Check sheet for the modelled part. Datum: model origin and axes. Units: mm. A direction names the side the tool comes from. Give positions to 0.01 mm unless a question says otherwise; leave off trailing zeros. Order: outer loops, then holes, each group sorted by start corner. A loop starts at its lowest first (then second) coordinate and runs counter-clockwise, first axis right, second up. Notation, with made-up numbers: (85.25, 30) -> (90.25, 30) arc R11 ccw to (90.25, 42) -> close; hole circle Ø5 at (58, 63). An arc over 180 degrees is marked (long way). One line per question, with ' | ' between items.
```python
from build123d import *

# Parameters (mm, degrees)
F1_DEPTH = 152.4
F2_DEPTH = 12.7
F3_R     = 3.175
F4_R     = 1.5875
F5_R     = 3.175
F6_DEPTH = 25.4


# Not quite as in the source:
# - a feature names something its author has since deleted; it is built from what else it names


with BuildPart() as f1:
    # F0 (on Top) → F1 (new body)
    with BuildSketch(Plane.XY):
        with BuildLine():
            Line((-6.35, 6.985), (10.6065911112, 6.985))
            ThreePointArc((10.6065911112, 6.985), (7.0295838714, 10.5770955652), (2.33256194, 12.4839558953))
            Line((2.33256194, 12.4839558953), (-6.35, 6.985))
        make_face()
        with BuildLine():
            ThreePointArc((2.33256194, 12.4839558953), (7.0295838714, 10.5770955652), (10.6065911112, 6.985))
            Line((10.6065911112, 6.985), (12.7, 6.985))
            Line((12.7, 6.985), (12.7, 13.2809655419))
            ThreePointArc((12.7, 13.2809655419), (11.0558438219, 16.0625374343), (7.8262096422, 15.9632661068))
            Line((7.8262096422, 15.9632661068), (2.33256194, 12.4839558953))
        make_face()
        with BuildLine():
            Line((12.7, -6.985), (10.6065911112, -6.985))
            ThreePointArc((10.6065911112, -6.985), (7.0295838714, -10.5770955652), (2.33256194, -12.4839558953))
            Line((2.33256194, -12.4839558953), (7.8262096422, -15.9632661068))
            ThreePointArc((7.8262096422, -15.9632661068), (11.0558438219, -16.0625374343), (12.7, -13.2809655419))
            Line((12.7, -13.2809655419), (12.7, -6.985))
        make_face()
        with BuildLine():
            ThreePointArc((2.33256194, -12.4839558953), (7.0295838714, -10.5770955652), (10.6065911112, -6.985))
            Line((10.6065911112, -6.985), (0, -6.985))
            Line((0, -6.985), (-6.35, -6.985))
            Line((-6.35, -6.985), (2.33256194, -12.4839558953))
        make_face()
        with BuildLine():
            Line((-6.35, 6.985), (2.33256194, 12.4839558953))
            ThreePointArc((2.33256194, 12.4839558953), (-8.1137680323, 9.7701979672), (-12.7, 0))
            Line((-12.7, 0), (-6.35, 0))
            Line((-6.35, 0), (-6.35, 6.985))
        make_face()
        with BuildLine():
            ThreePointArc((-10.6065911112, -6.985), (-4.9673452332, -11.6882625456), (2.33256194, -12.4839558953))
            Line((2.33256194, -12.4839558953), (-6.35, -6.985))
            Line((-6.35, -6.985), (-10.6065911112, -6.985))
        make_face()
        with BuildLine():
            Line((-6.35, 0), (-12.7, 0))
            ThreePointArc((-12.7, 0), (-12.1653957419, -3.6459767476), (-10.6065911112, -6.985))
            Line((-10.6065911112, -6.985), (-6.35, -6.985))
            Line((-6.35, -6.985), (-6.35, 0))
        make_face()
    extrude(amount=F1_DEPTH)

    # F0 (on Top) → F2 (join)
    with BuildSketch(Plane.XY):
        with BuildLine():
            Line((-6.35, 0), (-12.7, 0))
            ThreePointArc((-12.7, 0), (-12.1653957419, -3.6459767476), (-10.6065911112, -6.985))
            Line((-10.6065911112, -6.985), (-6.35, -6.985))
            Line((-6.35, -6.985), (-6.35, 0))
        make_face()
        with BuildLine():
            Line((-6.35, 6.985), (2.33256194, 12.4839558953))
            ThreePointArc((2.33256194, 12.4839558953), (-8.1137680323, 9.7701979672), (-12.7, 0))
            Line((-12.7, 0), (-6.35, 0))
            Line((-6.35, 0), (-6.35, 6.985))
        make_face()
        with BuildLine():
            ThreePointArc((-10.6065911112, -6.985), (-12.1653957419, -3.6459767476), (-12.7, 0))
            Line((-12.7, 0), (-25.4, 0))
            Line((-25.4, 0), (-25.4, -6.985))
            Line((-25.4, -6.985), (-10.6065911112, -6.985))
        make_face()
    extrude(amount=F2_DEPTH)

    # F3
    f3_edges = [f1.edges().sort_by_distance(p)[0] for p in [
        (-25.4, 0, 6.35),
        (-25.4, -6.985, 6.35),
    ]]
    fillet(f3_edges, radius=F3_R)

    # F4
    f4_edges = [f1.edges().sort_by_distance(p)[0] for p in [
        (-17.4625, 0, 12.7),
        (-24.470064, -0.929936, 12.7),
        (-25.4, -3.4925, 12.7),
        (-24.470064, -6.055064, 12.7),
        (-16.415796, -6.985, 12.7),
    ]]
    fillet(f4_edges, radius=F4_R)

    # F5 (on face) → F6 (cut)
    with BuildSketch(Plane(origin=(0, 0, 0), x_dir=(-1, 0, 0), z_dir=(0, 1, 0))):
        with Locations((17.4625, 5.55625)):
            Circle(F5_R)
    extrude(amount=-F6_DEPTH, mode=Mode.SUBTRACT)


solid = f1.part
```
Q1. Mould release check, pull along X, two halves, no side actions. Record for faces 1 (the face through (-20.395, -3.444, 4.34)), 2 (the face through (11.1, 16.04, 75.13)), 3 (the face through (0, 8, 152.4)): pulls with the +X half, pulls with the -X half, needs draft (parallel to the pull), parting line crosses it, or undercut.
Result sheet:
face 1: undercut | face 2: parting line crosses it | face 3: needs draft
Q2. Depth check by flat-ended pin: pin 1 Ø10 at (x, y) = (2, 9.5) entering from -Z; pin 2 Ø1.9 at (x, y) = (-15.5, -4) entering from +Z; pin 3 Ø12 at (x, z) = (-17.5, 5.5) entering from -Y (3 decimals); pin 4 Ø15 at (x, z) = (1.5, 46) entering from +Y. Enter the tip coordinate at first touch or a pass-through.
Result sheet:
pin 1: stops at z = 0 | pin 2: stops at z = 12.7 | pin 3: stops at y = -6.985 | pin 4: stops at y = 16.41
Q3. Section check C-C (x = -18.5). Enter the section's corners in (y, z) (1 decimal), and give its area (3 significant figures).
Result sheet:
outline: (-7, 0) -> (0, 0) -> (0, 2.6) -> (-7, 2.6) -> close; (-7, 8.6) -> (0, 8.6) -> (0, 11.1) arc R1.6 ccw to (-1.6, 12.7) -> (-5.4, 12.7) arc R1.6 ccw to (-7, 11.1) -> close | area: 45.7 mm2
Q4. Section check B-B (z = 110). Enter the section's corners in (x, y) (3 decimals), and give its area (3 significant figures).
Result sheet:
outline: (-6.35, -6.985) -> (-6.35, 6.985) -> (12.7, 6.985) -> (12.7, 13.281) arc R3.175 ccw to (7.826, 15.963) -> (2.333, 12.484) arc R12.7 ccw (long way) to (2.333, -12.484) -> (7.826, -15.963) arc R3.175 ccw to (12.7, -13.281) -> (12.7, -6.985) -> close | area: 358 mm2
Q5. Thickness scan on line 1 (Y direction, x = 0.5, z = 138) (3 decimals); line 2 (Y direction, x = 5, z = 36) (3 decimals); line 3 (X direction, y = 0.5, z = 40). Record the ranges inside material, lowest first.
Result sheet:
line 1: y = -12.69 to -6.985, 6.985 to 12.69 | line 2: y = -14.173 to -6.985, 6.985 to 14.173 | line 3: x = -12.69 to -6.35
Q6. Section check A-A (x = 4). Enter the section's corners in (y, z) (3 decimals), and give its area (3 significant figures).
Result sheet:
outline: (-13.54, 0) -> (-6.985, 0) -> (-6.985, 152.4) -> (-13.54, 152.4) -> close; (6.985, 0) -> (13.54, 0) -> (13.54, 152.4) -> (6.985, 152.4) -> close | area: 2,000 mm2
Q7. Section check D-D (y = 9). Enter the section's corners in (x, z), and give its area (3 significant figures).
Result sheet:
outline: (-8.96, 0) -> (12.7, 0) -> (12.7, 152.4) -> (-8.96, 152.4) -> close | area: 3,300 mm2
Q8. Access from +Z, -Z, +X, -X, +Y, -Y to the whole of each face (thin tool, end or side, straight path). Record for faces 4 (the face through (3, 6.985, 75)), 5 (the face through (-14, 0, 5)), 6 (the face through (-14, -6.985, 5)), 7 (the face through (12.7, 10, 75)).
Result sheet:
face 4: +Z, -Z, +X | face 5: +Z, -Z, -X, +Y | face 6: +Z, -Z, -X, -Y | face 7: +Z, -Z, +X, +Y, -Y
